Source: CAD feature listing. Evaluate the final solid. Frame: model axes, mm. Face numbers are marked on the shaded views. Round coordinates to 2 decimals unless told otherwise and drop trailing zeros. Write each loop counter-clockwise with the first axis right and the second up, starting at its lowest first coordinate (ties: lowest second). Pieces come first, ordered by that corner, then holes. Notation, with made-up numbers: M 76.25,46 L 92.25,46 A15 ccw 92.25,75 Z; hole C 60,-23 d4. An arc over 180 degrees is marked long. Use a Markdown table: item, result.
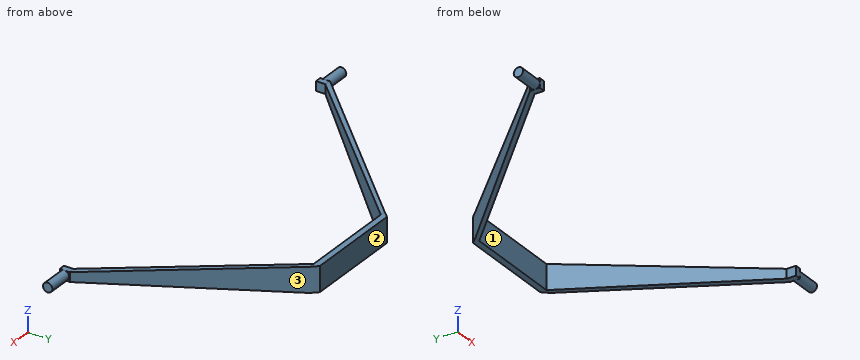
```python
from build123d import *

# Parameters (mm, degrees)
BOSS_EXTRUDE6_DEPTH            = 53.34
BOSS_EXTRUDE6_DEPTH_BACK       = 101.6
SKETCH13_R                     = 19.05
BOSS_EXTRUDE7_DEPTH            = 101.6
CUT_EXTRUDE8_REACH             = 992.358
CUT_EXTRUDE8_DIRECTION_2_REACH = 992.358


with BuildPart() as part:
    # Sketch12 → Boss-Extrude6 (new, two sides: drawn at the far end of the back side and taken through both)
    with BuildSketch(Plane.XY.offset(-BOSS_EXTRUDE6_DEPTH_BACK)):
        Polygon((-203.2, 241.3), (203.2, 241.3), (787.471663752, -383.669201703), (787.471663752, -424.309201703), (762.071663752, -424.309201703), (762.071663752, -386.209201703), (203.2, 215.9), (-203.2, 215.9), (-762.071663752, -386.209201703), (-762.071663752, -424.309201703), (-787.471663752, -424.309201703), (-787.471663752, -383.669201703), align=None)
    extrude(amount=BOSS_EXTRUDE6_DEPTH + BOSS_EXTRUDE6_DEPTH_BACK)

    # Sketch13 → Boss-Extrude7 (add)
    with BuildSketch(Plane(origin=(787.471663752, 0, 0), x_dir=(0, 0, -1), z_dir=(1, 0, 0))):
        with Locations(Location((-34.29, -405.259201703, 0), (0, 0, 180))):
            Circle(SKETCH13_R)
    boss_extrude7 = extrude(amount=BOSS_EXTRUDE7_DEPTH)

    # Mirror1: Boss-Extrude7 across plane
    add(boss_extrude7.mirror(Plane(origin=(0, 0, 0), x_dir=(0, 0, 1), z_dir=(1, 0, 0))))

    # Cut-Extrude8: up to this plane
    cut_extrude8_end = Plane(origin=(-203.2, 241.3, -101.6), z_dir=(-0.7304911811601322, 0.6829221289775833, 0))
    # Sketch14 → Cut-Extrude8 (cut, up to the surface)
    with BuildSketch(Plane(origin=(0, 0, 0), x_dir=(0, 0, -1), z_dir=(1, 0, 0)), mode=Mode.PRIVATE) as cut_extrude8_sk1:
        Polygon((0, 241.3), (0, 215.9), (-53.34, -386.209201703), (-53.34, 241.3), align=None)
    cut_extrude8_tool1 = split(extrude(cut_extrude8_sk1.sketch, amount=-CUT_EXTRUDE8_REACH, mode=Mode.PRIVATE), bisect_by=cut_extrude8_end, keep=Keep.BOTH, mode=Mode.PRIVATE)
    add(cut_extrude8_tool1.solids().sort_by_distance((0, 31.800889, 34.868308))[0], mode=Mode.SUBTRACT)
    # Sketch14 → Cut-Extrude8 (cut, up to the surface)
    with BuildSketch(Plane(origin=(0, 0, 0), x_dir=(0, 0, -1), z_dir=(1, 0, 0)), mode=Mode.PRIVATE) as cut_extrude8_sk2:
        Polygon((101.6, 215.9), (-15.24, -386.209201703), (-15.24, -424.309201703), (101.6, -424.309201703), align=None)
    cut_extrude8_tool2 = split(extrude(cut_extrude8_sk2.sketch, amount=-CUT_EXTRUDE8_REACH, mode=Mode.PRIVATE), bisect_by=cut_extrude8_end, keep=Keep.BOTH, mode=Mode.PRIVATE)
    add(cut_extrude8_tool2.solids().sort_by_distance((0, -210.192787, -60.465735))[0], mode=Mode.SUBTRACT)

    # Cut-Extrude8 direction 2: up to this plane
    cut_extrude8_direction_2_end = Plane(origin=(203.2, 241.3, -101.6), z_dir=(0.7304911811601321, 0.6829221289775835, 0))
    # Sketch14 → Cut-Extrude8 direction 2 (cut, up to the surface)
    with BuildSketch(Plane(origin=(0, 0, 0), x_dir=(0, 0, -1), z_dir=(1, 0, 0)), mode=Mode.PRIVATE) as cut_extrude8_direction_2_sk1:
        Polygon((0, 241.3), (0, 215.9), (-53.34, -386.209201703), (-53.34, 241.3), align=None)
    cut_extrude8_direction_2_tool1 = split(extrude(cut_extrude8_direction_2_sk1.sketch, amount=CUT_EXTRUDE8_DIRECTION_2_REACH, mode=Mode.PRIVATE), bisect_by=cut_extrude8_direction_2_end, keep=Keep.BOTH, mode=Mode.PRIVATE)
    add(cut_extrude8_direction_2_tool1.solids().sort_by_distance((0, 31.800889, 34.868308))[0], mode=Mode.SUBTRACT)
    # Sketch14 → Cut-Extrude8 direction 2 (cut, up to the surface)
    with BuildSketch(Plane(origin=(0, 0, 0), x_dir=(0, 0, -1), z_dir=(1, 0, 0)), mode=Mode.PRIVATE) as cut_extrude8_direction_2_sk2:
        Polygon((101.6, 215.9), (-15.24, -386.209201703), (-15.24, -424.309201703), (101.6, -424.309201703), align=None)
    cut_extrude8_direction_2_tool2 = split(extrude(cut_extrude8_direction_2_sk2.sketch, amount=CUT_EXTRUDE8_DIRECTION_2_REACH, mode=Mode.PRIVATE), bisect_by=cut_extrude8_direction_2_end, keep=Keep.BOTH, mode=Mode.PRIVATE)
    add(cut_extrude8_direction_2_tool2.solids().sort_by_distance((0, -210.192787, -60.465735))[0], mode=Mode.SUBTRACT)


solid = part.part
```
Q1. Line query: L1, parallel to Y at x = 10, z = -93.5; L2, parallel to X at y = 210, z = -5.5; L3, parallel to X at y = 38, z = -66. Output: solid intervals per line, ascending.
Results are:
| item | result |
|---|---|
| L1 | 215.9 to 241.3 |
| L2 | -232.46 to -208.68, 208.68 to 232.46 |
| L3 | -393.26 to -368.32, 368.32 to 393.26 |
Q2. First-contact query: pin 1 Ø7.5 at (x, y) = (86, 229.5) entering from +Z; pin 2 Ø10 at (x, z) = (-23, -12.5) entering from -Y; pin 3 Ø4 at (y, z) = (140, -45.5) entering from +X. Flat tips, straight axial feed; report the tip coordinate or a pass-through.
Results are:
| item | result |
|---|---|
| pin 1 | z = 0 |
| pin 2 | y = 215.9 |
| pin 3 | x = 299.77 |
Q3. Mould query, pull axis X, two halves, no side actions, for the marked faces 1, 2 and 3. Classes: +X half, -X half, draft (parallel to the pull), parting line (faces both ways), or undercut.
Results are:
| item | result |
|---|---|
| face 1 | undercut |
| face 2 | draft |
| face 3 | +X half |
Q4. Section A-A on y = -178.5. Return loops of the section in (x, z), plus the area to 3 significant figures.
Results are:
| item | result |
|---|---|
| outline | M -595.66,-25.07 L -569.28,-25.07 L -569.28,34.94 L -595.66,34.94 Z; M 569.28,-25.07 L 595.66,-25.07 L 595.66,34.94 L 569.28,34.94 Z |
| area | 3,170 mm^2 |
Q5. Section C-C on y = -329. Return loops of the section in (x, z), plus the area to 3 significant figures.
Results are:
| item | result |
|---|---|
| outline | M -736.36,4.14 L -708.97,4.14 L -708.97,48.27 L -736.36,48.27 Z; M 708.97,4.14 L 736.36,4.14 L 736.36,48.27 L 708.97,48.27 Z |
| area | 2,420 mm^2 |
Q6. Section B-B on z = -71.5. Return loops of the section in (x, y).
Results are:
| item | result |
|---|---|
| outline | M -371.96,60.79 L -347.17,60.79 L -203.2,215.9 L 203.2,215.9 L 347.17,60.79 L 371.96,60.79 L 203.2,241.3 L -203.2,241.3 Z |
Q7. Section D-D on x = -177.5. Return loops of the section in (y, z), plus the area to 3 significant figures.
Results are:
| item | result |
|---|---|
| outline | M 215.9,-101.6 L 241.3,-101.6 L 241.3,0 L 215.9,0 Z |
| area | 2,580 mm^2 |
